Could you check a few things on this model? Use its own coordinates, in mm. Face numbers are marked on the shaded views. A direction names the side the tool comes from. Coordinates: 2 decimals unless noted, no trailing zeros. Write each loop counter-clockwise with the first axis right and the second up, starting at its lowest first coordinate (ties: lowest second). Pieces come first, ordered by that corner, then holes.
```python
from build123d import *

# Parameters (mm, degrees)
BOSS_EXTRUDE1_DEPTH = 12
FILLET1_R           = 6
SKETCH2_R           = 3.15
CUT_EXTRUDE1_DEPTH  = 70
CUT_EXTRUDE2_START  = -12
SKETCH3_R           = 5
CUT_EXTRUDE2_DEPTH  = 3.5
SKETCH3_3_R         = 1.45
CUT_EXTRUDE3_DEPTH  = 13.5
SKETCH3_4_R         = 2.6
CUT_EXTRUDE4_DEPTH  = 4.4
SKETCH3_5_R         = 5
CUT_EXTRUDE5_DEPTH  = 3.5
SKETCH3_6_R         = 1.45
CUT_EXTRUDE6_DEPTH  = 18
CUT_EXTRUDE7_START  = -12
SKETCH3_7_R         = 2.6
CUT_EXTRUDE7_DEPTH  = 4.4


with BuildPart() as part:
    # Sketch1 → Boss-Extrude1 (new body)
    with BuildSketch(Plane(origin=(0, 0, 0), x_dir=(1, 0, 0), z_dir=(0, 1, 0))):
        with BuildLine():
            ThreePointArc((-40, -6), (-23.323807589, -23.539679293), (-2.2e-08, -30))
            ThreePointArc((-2.2e-08, -30), (23.32380757, -23.539679305), (40, -6))
            Line((40, -6), (40, 17))
            Line((40, 17), (24, 17))
            Line((24, 17), (24, 30))
            Line((24, 30), (-24, 30))
            Line((-24, 30), (-24, 17))
            Line((-24, 17), (-40, 17))
            Line((-40, 17), (-40, -6))
        make_face()
    extrude(amount=BOSS_EXTRUDE1_DEPTH)

    # Fillet1
    fillet1_edges = [part.edges().sort_by_distance(p)[0] for p in [
        (0, 0, -30),
        (0, 12, -30),
    ]]
    fillet(fillet1_edges, radius=FILLET1_R - 0.0001)  # a hair under: the kernel refuses the full size

    # Sketch2 → Cut-Extrude1 (cut)
    with BuildSketch(Plane.ZY.offset(24)):
        with Locations((-24, 6)):
            Circle(SKETCH2_R)
    extrude(amount=-CUT_EXTRUDE1_DEPTH, mode=Mode.SUBTRACT)

    # Sketch3 → Cut-Extrude2 (cut)
    with BuildSketch(Plane(origin=(0, 12, 0), x_dir=(1, 0, 0), z_dir=(0, 1, 0)).offset(CUT_EXTRUDE2_START)):
        with Locations(Location((-12, 17, 0), (0, 0, 270))):
            Circle(SKETCH3_R)
    extrude(amount=CUT_EXTRUDE2_DEPTH, mode=Mode.SUBTRACT)

    # Sketch3<3> → Cut-Extrude3 (cut)
    with BuildSketch(Plane(origin=(0, 12, 0), x_dir=(1, 0, 0), z_dir=(0, 1, 0))):
        with Locations(Location((-12, 17, 0), (0, 0, 270))):
            Circle(SKETCH3_3_R)
    extrude(amount=-CUT_EXTRUDE3_DEPTH, mode=Mode.SUBTRACT)

    # Sketch3<4> → Cut-Extrude4 (cut)
    with BuildSketch(Plane(origin=(0, 12, 0), x_dir=(1, 0, 0), z_dir=(0, 1, 0))):
        with Locations(Location((-12, 17, 0), (0, 0, 270))):
            Circle(SKETCH3_4_R)
    extrude(amount=-CUT_EXTRUDE4_DEPTH, mode=Mode.SUBTRACT)

    # Sketch3<5> → Cut-Extrude5 (cut)
    with BuildSketch(Plane(origin=(0, 12, 0), x_dir=(1, 0, 0), z_dir=(0, 1, 0))):
        with Locations(Location((12, 17, 0), (0, 0, 270))):
            Circle(SKETCH3_5_R)
    extrude(amount=-CUT_EXTRUDE5_DEPTH, mode=Mode.SUBTRACT)

    # Sketch3<6> → Cut-Extrude6 (cut)
    with BuildSketch(Plane(origin=(0, 12, 0), x_dir=(1, 0, 0), z_dir=(0, 1, 0))):
        with Locations(Location((12, 17, 0), (0, 0, 270))):
            Circle(SKETCH3_6_R)
    extrude(amount=-CUT_EXTRUDE6_DEPTH, mode=Mode.SUBTRACT)

    # Sketch3<7> → Cut-Extrude7 (cut)
    with BuildSketch(Plane(origin=(0, 12, 0), x_dir=(1, 0, 0), z_dir=(0, 1, 0)).offset(CUT_EXTRUDE7_START)):
        with Locations(Location((12, 17, 0), (0, 0, 270))):
            Circle(SKETCH3_7_R)
    extrude(amount=CUT_EXTRUDE7_DEPTH, mode=Mode.SUBTRACT)


solid = part.part
```
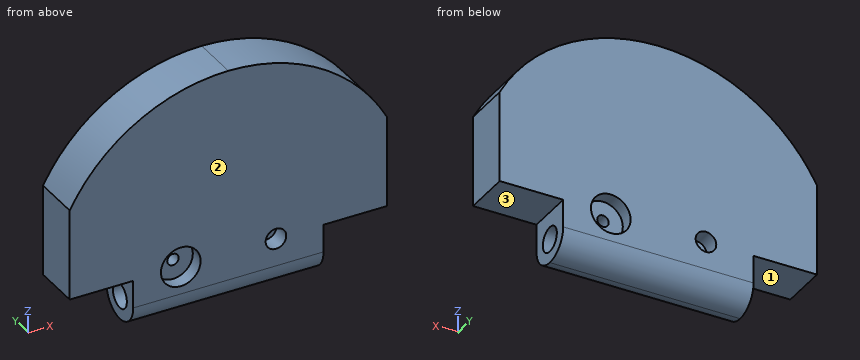
1. I want a section at B-B on y = 1. Please give me the cut outline in (x, z), plus the area to 3 significant figures.
Verdict:
outline: (-40, -17) - (-24, -17) - (-24, -27.32) - (24, -27.32) - (24, -17) - (40, -17) - (40, 6) arc R45.33 ccw to (-40, 6) - close; hole circle Ø10 at (-12, -17); hole circle Ø5.2 at (12, -17)
area: 3,600 mm2
2. I want a section at A-A on x = 12. Give the number of separate pieces and of enclosed holes in the cut face, plus the area to 3 significant figures.
Verdict:
separate pieces: 2
enclosed holes: 1
area: 584 mm2
3. I want a section at C-C on z = 12. Please give me the cut outline in (x, y), plus the area to 3 significant figures.
Verdict:
outline: (-36.17, 0) - (36.17, 0) - (36.17, 12) - (-36.17, 12) - close
area: 868 mm2
4. I want a section at D-D on x = 33.5. Please give me the cut outline in (y, z), plus the area to 3 significant figures.
Verdict:
outline: (0, -17) - (12, -17) - (12, 15.21) - (0, 15.21) - close
area: 387 mm2
5. Please list where these lines run through material, in increasing order: line 1 along Y through (x, z) = (-10, -18); line 2 along Z through (x, y) = (-18.5, 3.25); line 3 along Z through (x, y) = (13.5, 2).
Verdict:
line 1: y = 3.5 to 7.6
line 2: z = -29.33 to -25.54, -22.46 to 26.05
line 3: z = -28.47 to -19.12, -14.88 to 27.94
6. For pin 1 (1.6 mm diameter, centred on x = 12.5, z = -18, fed in from -Y); pin 2 (7 mm diameter, centred on y = 6, z = -24, fed in from +X); pin 3 (1 mm diameter, centred on x = 25, y = 9, fed in from +Z); pin 4 (1.6 mm diameter, centred on x = -11.5, z = -17, fed in from +Y), each with a flat end and sliding along its axis, tell me the tip position at first contact or that it passes through.
Verdict:
pin 1: stops at y = 4.4
pin 2: stops at x = 24
pin 3: stops at z = 22.81
pin 4: passes through
7. On a 3-axis mill with a long thin cutter (end or side, diameter ignored), from which of +Z, -Z, +X, -X, +Y, -Y can I reach the whole of each face in a straight line? I mean the marked faces 1, 2 and 3. Say none if no direction works.
Verdict:
face 1: -Z, -X, +Y, -Y
face 2: +Z, -Z, +X, -X, -Y
face 3: -Z, +X, +Y, -Y
